Check sheet for the modelled part. Datum: model origin and axes. Units: mm. Face numbers are marked on the shaded views. A direction names the side the tool comes from. Coordinates: 2 decimals unless noted, no trailing zeros. Loops run counter-clockwise (first coordinate to the right, second up) from the corner with the lowest first, then second, coordinate; pieces in that order, holes last. Notation, with made-up numbers: (-10.5, 56) -> (16.5, 56) arc R17 cw to (16.5, 74) -> close; hole circle Ø6 at (-7.5, 5). An arc over 180 degrees is marked (long way). Use CSV: the item, a comma, the result in double quotes.
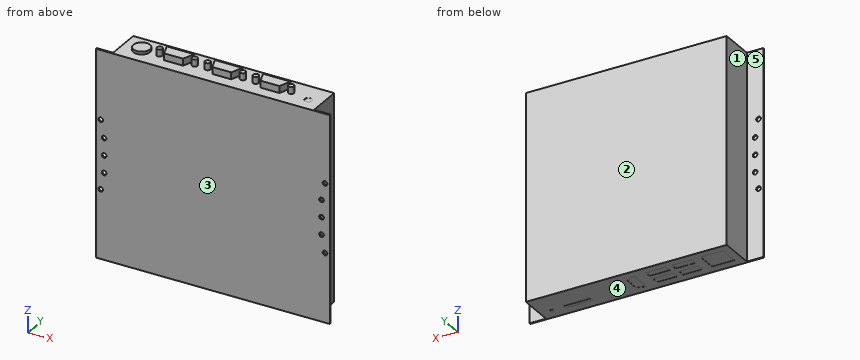
```python
from build123d import *

# Parameters (mm, degrees)
SKETCH_1_W             = 146
SKETCH_1_H             = 150
EXTRUDE_1_DEPTH        = 26
SKETCH_2_W             = 170
SKETCH_2_H             = 150
EXTRUDE_2_DEPTH        = 1
HOLE_WIZARD_M3_1_D     = 3.4
SKETCH_5_R             = 6.063811431
EXTRUDE_3_DEPTH        = 2
SKETCH_6_R             = 2.017692423
SKETCH_6_R_2           = 2.03992662
EXTRUDE_4_DEPTH        = 5
PATTERN_LINEAR_1_COUNT = 3
PATTERN_LINEAR_1_PITCH = 35
SKETCH_7_R             = 2.600130351
CUT_EXTRUDE_1_DEPTH    = 0.1
SKETCH_8_W             = 14.672164123
SKETCH_8_H             = 4.828813509
SKETCH_8_W_2           = 14.114993332
SKETCH_8_H_2           = 5.014537105
SKETCH_8_W_3           = 16.157952894
SKETCH_8_H_3           = 14.114993333
CUT_EXTRUDE_2_DEPTH    = 0.1
SKETCH_9_R             = 1.296267094
SKETCH_9_W             = 20.070729893
SKETCH_9_H             = 2.548664114
EXTRUDE_5_DEPTH        = 0.1


with BuildPart() as part:
    # 草图1 → 凸台-拉伸1 (new body)
    with BuildSketch(Plane(origin=(0, 0, 0), x_dir=(1, 0, 0), z_dir=(0, 1, 0))):
        Rectangle(SKETCH_1_W, SKETCH_1_H)
    extrude(amount=EXTRUDE_1_DEPTH)

    # 草图2 → 凸台-拉伸2 (add)
    with BuildSketch(Plane.XZ):
        Rectangle(SKETCH_2_W, SKETCH_2_H)
    extrude(amount=-EXTRUDE_2_DEPTH)

    # M3 间隙孔1 (through all)
    with Locations(Plane(origin=(0, 1, 0), x_dir=(1, 0, 0), z_dir=(0, 1, 0))):
        with Locations((-81.5, 25), (-81.5, -25), (81.5, 25), (81.5, -25), (-79, 12.5), (-79, 0), (-79, -12.5), (79, -12.5), (79, 0), (79, 12.5)):
            Hole(HOLE_WIZARD_M3_1_D / 2)

    # 草图5 → 凸台-拉伸3 (add)
    with BuildSketch(Plane.XY.offset(75)):
        with Locations(Location((-59.431550874, 13.278585395, 0), (0, 0, 180))):
            Circle(SKETCH_5_R)
    extrude(amount=EXTRUDE_3_DEPTH)

    # 草图6 → 凸台-拉伸4 (add)
    with BuildSketch(Plane.XY.offset(75)):
        with Locations(Location((-46.32884835, 13.11494848, 0), (0, 0, 180))):
            Circle(SKETCH_6_R)
        with Locations(Location((-20.769548413, 13.11494848, 0), (0, 0, 180))):
            Circle(SKETCH_6_R_2)
        Polygon((-43.590070032, 17.274031542), (-23.590070032, 17.274031542), (-26.696119877, 8.72468841), (-40.484020187, 8.72468841), align=None)
    extrude_4 = extrude(amount=EXTRUDE_4_DEPTH)

    # 阵列(线性)1: 凸台-拉伸4 ×3
    with Locations(*[(i * PATTERN_LINEAR_1_PITCH, 0, 0) for i in range(1, PATTERN_LINEAR_1_COUNT)]):
        add(extrude_4)

    # 草图7 → 切除-拉伸1 (cut)
    with BuildSketch(Plane.XY.offset(75)):
        with Locations((63.517469997, 10.121284255)):
            Circle(SKETCH_7_R)
    extrude(amount=-CUT_EXTRUDE_1_DEPTH, mode=Mode.SUBTRACT)

    # 草图8 → 切除-拉伸2 (cut)
    with BuildSketch(Plane(origin=(0, 0, -75), x_dir=(-1, 0, 0), z_dir=(0, 0, -1))):
        Polygon((2.600130351, 20.521805658), (-4.085919123, 17.995663664), (-4.085919123, 7.154283691), (2.600130351, 4.921023553), align=None)
        with Locations((18.293774254, 18.107398904)):
            Rectangle(SKETCH_8_W, SKETCH_8_H)
        with Locations((36.9589957, 18.107398904)):
            Rectangle(SKETCH_8_W_2, SKETCH_8_H)
        with Locations((18.293774254, 8.914080878)):
            Rectangle(SKETCH_8_W, SKETCH_8_H_2)
        with Locations((36.9589957, 8.914080878)):
            Rectangle(SKETCH_8_W_2, SKETCH_8_H_2)
        with Locations((58.967241883, 13.464308992)):
            Rectangle(SKETCH_8_W_3, SKETCH_8_H_3)
    extrude(amount=-CUT_EXTRUDE_2_DEPTH, mode=Mode.SUBTRACT)

    # 草图9 → 凸台-拉伸5 (add)
    with BuildSketch(Plane(origin=(0, 0, -75), x_dir=(-1, 0, 0), z_dir=(0, 0, -1))):
        with Locations(Location((-64.611587391, 7.936618922, 0), (0, 0, 180))):
            Circle(SKETCH_9_R)
        with Locations((-45.443509371, 8.149007598)):
            Rectangle(SKETCH_9_W, SKETCH_9_H)
    extrude(amount=EXTRUDE_5_DEPTH)


solid = part.part
```
1) Cross-section at A-A on z = -46. Record the boundary of the cut face in (x, y).
Answer below:
outline,"(-85, 0) -> (85, 0) -> (85, 1) -> (73, 1) -> (73, 26) -> (-73, 26) -> (-73, 1) -> (-85, 1) -> close"
2) Draft check along Y on the marked faces 3, 4 and 5. Enter one of: released by +Y, released by -Y, zero draft, split by the parting line, or undercut.
Answer below:
face 3,"released by -Y"
face 4,"zero draft"
face 5,"released by +Y"
3) Access from +Z, -Z, +X, -X, +Y, -Y to the whole of each face (thin tool, end or side, straight path). Record for the marked faces 1 and 2.
Answer below:
face 1,"+Z, -Z, -X, +Y"
face 2,"+Z, -Z, +X, -X, +Y"
4) Go/stop test with flat-tipped pins: pin 1 Ø8 at (y, z) = (22, 10) entering from -X; pin 2 Ø8 at (x, z) = (-44, -6.5) entering from -Y; pin 3 Ø4 at (x, y) = (-57.5, 10.5) entering from -Z; pin 4 Ø3 at (x, y) = (-9.5, 21) entering from +Z. Record where each tip stops, or that it passes through.
Answer below:
pin 1,"stops at x = -73"
pin 2,"stops at y = 0"
pin 3,"stops at z = -74.9"
pin 4,"stops at z = 75"
5) Thickness scan on line 1 along Z through (x, y) = (-81.5, 0.85); line 2 along X through (y, z) = (0.2, 25); line 3 along Z through (x, y) = (79, 0.65). Record the ranges inside material, lowest first. Write a range as from..to.
Answer below:
line 1,"z = -75..-26.7, -23.3..23.3, 26.7..75"
line 2,"x = -85..-83.2, -79.8..79.8, 83.2..85"
line 3,"z = -75..-14.2, -10.8..-1.7, 1.7..10.8, 14.2..75"
6) Cross-section at B-B on x = -57. Record the boundary of the cut face in (y, z), and give its area (3 significant figures).
Answer below:
outline,"(0, -75) -> (6.41, -75) -> (6.41, -74.9) -> (20.52, -74.9) -> (20.52, -75) -> (26, -75) -> (26, 75) -> (18.83, 75) -> (18.83, 77) -> (7.72, 77) -> (7.72, 75) -> (0, 75) -> close"
area,"3,920 mm²"
